Verification items for the finished model (mm, model axes). Face numbers are marked on the shaded views. A direction names the side the tool comes from. Coordinates: 2 decimals unless noted, no trailing zeros. Order: outer loops, then holes, each group sorted by start corner. A loop starts at its lowest first (then second) coordinate and runs counter-clockwise, first axis right, second up. Notation, with made-up numbers: (36.5, 76.25) -> (87.5, 76.25) arc R35 ccw to (87.5, 108.25) -> close; hole circle Ø6 at (38.25, 0). An arc over 180 degrees is marked (long way). Write item = value, one per line. Start each with the question number.
1. Cross-section at D-D on z = -6.75. Record the cut outline in (x, y), plus the area to 3 significant figures.
2. Go/stop test with flat-tipped pins: P1, Ø3.5, axis at x = 15, z = 0, coming from the -Y side; P2, Ø12, axis at y = 21, z = 2, coming from the +X side. Record where each tip stops, or that it passes through.
3. Cross-section at A-A on x = 15. Record the cut outline in (y, z), plus the area to 3 significant figures.
4. Set-up check for the marked faces 1 and 2: record each of +Z, -Z, +X, -X, +Y, -Y from which the full face is reachable in a straight line by a thin tool's end or side.
5. Thickness scan on line 1 along Y through (x, z) = (1.2, 0); line 2 along Y through (x, z) = (25.5, -3.5). Record the ranges inside material, lowest first. Write a range as from..to.
6. Cross-section at B-B on z = 0. Record the cut outline in (x, y), plus the area to 3 significant figures.
7. Release check for a two-part mould opening along Y. For the marked faces 3, 4, 5 and 6 record: +Y half, -Y half, draft (parallel to the pull), parting line (faces both ways), or undercut.
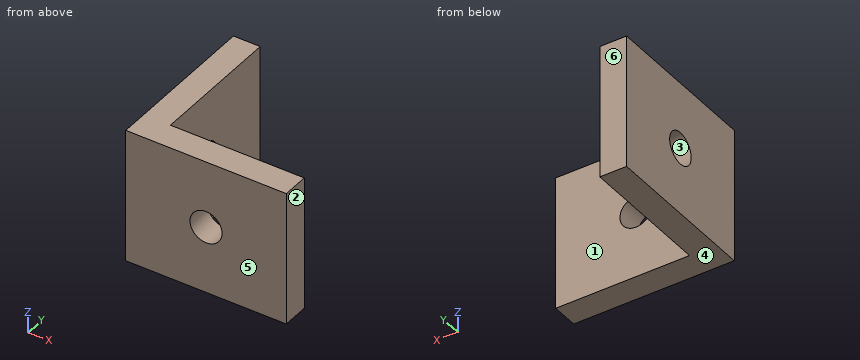
from build123d import *

# Parameters (mm, degrees)
BOSS_EXTRUDE1_DEPTH = 12.5
SKETCH2_R           = 3
CUT_EXTRUDE1_DEPTH  = 45.229515032
SKETCH3_R           = 3
CUT_EXTRUDE2_DEPTH  = 45.229515032


with BuildPart() as part:
    # Sketch1 → Boss-Extrude1 (new, symmetric)
    with BuildSketch(Plane.XY):
        Polygon((0, 0), (0, 30), (5, 30), (5, 5), (30, 5), (30, 0), align=None)
    extrude(amount=BOSS_EXTRUDE1_DEPTH, both=True)

    # Sketch2 → Cut-Extrude1 (cut, through all)
    with BuildSketch(Plane.ZY):
        with Locations((0, 15)):
            Circle(SKETCH2_R)
    extrude(amount=-CUT_EXTRUDE1_DEPTH, mode=Mode.SUBTRACT)

    # Sketch3 → Cut-Extrude2 (cut, through all)
    with BuildSketch(Plane(origin=(0, 0, 0), x_dir=(0, 0, 1), z_dir=(0, -1, 0))):
        with Locations(Location((0, -15, 0), (0, 0, 270))):
            Circle(SKETCH3_R)
    extrude(amount=-CUT_EXTRUDE2_DEPTH, mode=Mode.SUBTRACT)


solid = part.part
Worked out:
q1.outline = (0, 0) -> (30, 0) -> (30, 5) -> (5, 5) -> (5, 30) -> (0, 30) -> close
q1.area = 275 mm²
q2.P1 = through
q2.P2 = 5
q3.outline = (0, -12.5) -> (5, -12.5) -> (5, -3) -> (0, -3) -> close; (0, 3) -> (5, 3) -> (5, 12.5) -> (0, 12.5) -> close
q3.area = 95.0 mm²
q4.face_1 = +Z, -Z, +X, +Y
q4.face_2 = +Z, -Z, +X, +Y, -Y
q5.line_1 = 0..12, 18..30
q5.line_2 = 0..5
q6.outline = (0, 0) -> (12, 0) -> (12, 5) -> (5, 5) -> (5, 12) -> (0, 12) -> close; (0, 18) -> (5, 18) -> (5, 30) -> (0, 30) -> close; (18, 0) -> (30, 0) -> (30, 5) -> (18, 5) -> close
q6.area = 215 mm²
q7.face_3 = undercut
q7.face_4 = draft
q7.face_5 = -Y half
q7.face_6 = +Y half
